Geometry check sheet. Reference: the model listing, model coordinates, mm. Round coordinates to 2 decimals unless told otherwise and drop trailing zeros. Write each loop counter-clockwise with the first axis right and the second up, starting at its lowest first coordinate (ties: lowest second). Pieces come first, ordered by that corner, then holes. Notation, with made-up numbers: (62, 42.5) -> (120, 42.5) arc R24 cw to (120, 53.5) -> close; hole circle Ø8 at (27.25, -14.75). An arc over 180 degrees is marked (long way). Use a Markdown table: item, result.
```python
from build123d import *

# Parameters (mm, degrees)
EXTRUDE_1_DEPTH   = 2
HOLE_WIZARD_M81_D = 9
CHAMFER_1_SIZE    = 2


with BuildPart() as part:
    # Эскиз1 → Бобышка-Вытянуть1 (new body)
    with BuildSketch(Plane(origin=(0, 0, 0), x_dir=(1, 0, 0), z_dir=(0, 0, -1))):
        Polygon((0, 0), (0, 90), (90, 90), (90, 45), (45, 0), align=None)
    extrude(amount=EXTRUDE_1_DEPTH)

    # Отверстие с зазором M81 (through all)
    with Locations(Plane(origin=(0, 0, -2), x_dir=(1, 0, 0), z_dir=(0, 0, -1))):
        with Locations((22.5, 67.5), (22.5, 22.5), (67.5, 67.5)):
            Hole(HOLE_WIZARD_M81_D / 2)

    # Фаска1
    chamfer_1_edges = [part.edges().sort_by_distance(p)[0] for p in [
        (0, 0, -1),
        (0, -90, -1),
        (90, -90, -1),
    ]]
    chamfer(chamfer_1_edges, length=CHAMFER_1_SIZE)


solid = part.part
```
(1) Gauge pin test, flat end, axial feed: pin 1 Ø11.5 at (x, y) = (22.5, -22.5) entering from -Z. Record the tip position at first contact, or that the pin passes through.
A:
| item | result |
|---|---|
| pin 1 | stops at z = -2 |
(2) Section check C-C on z = -1.2. Record the cut outline in (x, y).
A:
| item | result |
|---|---|
| outline | (0, -88) -> (2, -90) -> (88, -90) -> (90, -88) -> (90, -45) -> (45, 0) -> (2, 0) -> (0, -2) -> close; hole circle Ø9 at (22.5, -67.5); hole circle Ø9 at (22.5, -22.5); hole circle Ø9 at (67.5, -67.5) |
(3) Section check D-D on x = 22.5. Record the cut outline in (y, z), plus the area to 3 significant figures.
A:
| item | result |
|---|---|
| outline | (-90, -2) -> (-72, -2) -> (-72, 0) -> (-90, 0) -> close; (-63, -2) -> (-27, -2) -> (-27, 0) -> (-63, 0) -> close; (-18, -2) -> (0, -2) -> (0, 0) -> (-18, 0) -> close |
| area | 144 mm2 |
(4) Thickness scan on line 1 (X direction, y = -67.5, z = -1.45); line 2 (Y direction, x = 22.5, z = -1.6); line 3 (X direction, y = -65, z = -1.9). Record the ranges inside material, lowest first.
A:
| item | result |
|---|---|
| line 1 | x = 0 to 18, 27 to 63, 72 to 90 |
| line 2 | y = -90 to -72, -63 to -27, -18 to 0 |
| line 3 | x = 0 to 18.76, 26.24 to 63.76, 71.24 to 90 |
(5) Section check B-B on y = -22.5. Record the cut outline in (x, z).
A:
| item | result |
|---|---|
| outline | (0, -2) -> (18, -2) -> (18, 0) -> (0, 0) -> close; (27, -2) -> (67.5, -2) -> (67.5, 0) -> (27, 0) -> close |
(6) Section check A-A on x = 67.5. Record the cut outline in (y, z), plus the area to 3 significant figures.
A:
| item | result |
|---|---|
| outline | (-90, -2) -> (-72, -2) -> (-72, 0) -> (-90, 0) -> close; (-63, -2) -> (-22.5, -2) -> (-22.5, 0) -> (-63, 0) -> close |
| area | 117 mm2 |
